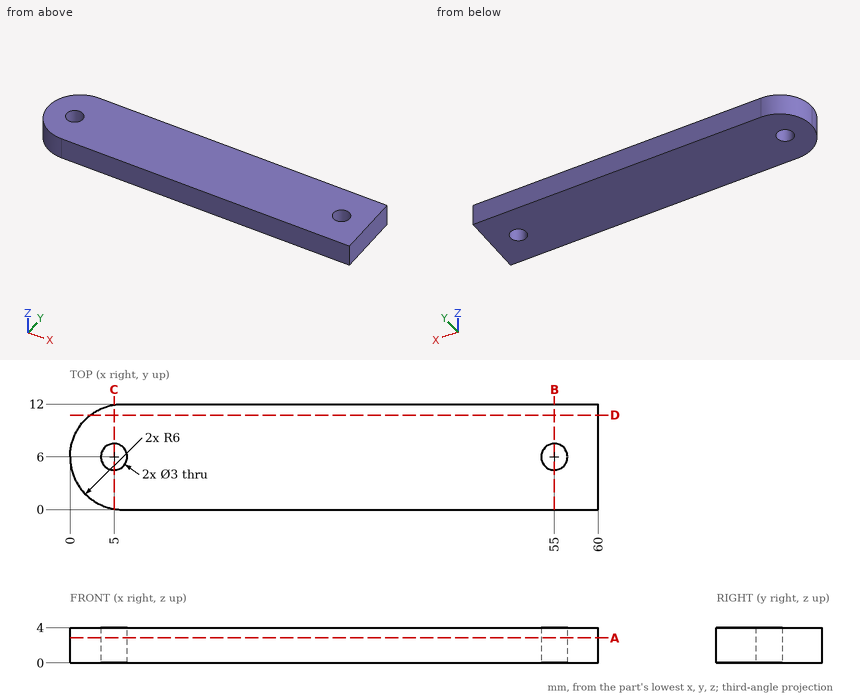
Here's the drawing with two shaded views (mm, measured from the low corner). I have some questions. Coordinates: 2 decimals unless noted, no trailing zeros. Write each loop counter-clockwise with the first axis right and the second up, starting at its lowest first coordinate (ties: lowest second). Pieces come first, ordered by that corner, then holes. Notation, with made-up numbers: (16, -2) -> (55, -2) arc R23 ccw to (55, 35) -> close; hole circle Ø11 at (37, -23.75). An arc over 180 degrees is marked (long way). One line per question, with ' | ' between items. Start each with the question number.
1. If we section it at C-C (x = 5): Please give me the cut outline in (y, z), and give its area (3 significant figures).
2. If we section it at B-B (x = 55): Please give me the cut outline in (y, z), and give its area (3 significant figures).
3. Please list where these lines run through material, in increasing order: line 1 along Y through (x, z) = (55, 2.5); line 2 along X through (y, z) = (5, 3.5); line 3 along Y through (x, z) = (6, 2.85).
4. Will this pin go through, and if not, where does the flat tip stop? P1, Ø2, axis at y = 9.5, z = 1.5, coming from the -X side.
5. If we section it at A-A (z = 2.85): Count the separate pieces of the cut face and the enclosed holes in it, and give its area (3 significant figures).
6. If we section it at D-D (y = 10.75): Please give me the cut outline in (x, z), and give its area (3 significant figures).
Return value:
1) outline: (0.08, 0) -> (4.5, 0) -> (4.5, 4) -> (0.08, 4) -> close; (7.5, 0) -> (11.92, 0) -> (11.92, 4) -> (7.5, 4) -> close | area: 35.3 mm²
2) outline: (0, 0) -> (4.5, 0) -> (4.5, 4) -> (0, 4) -> close; (7.5, 0) -> (12, 0) -> (12, 4) -> (7.5, 4) -> close | area: 36.0 mm²
3) line 1: y = 0 to 4.5, 7.5 to 12 | line 2: x = 0.08 to 3.88, 6.12 to 53.88, 56.12 to 60 | line 3: y = 0 to 4.88, 7.12 to 12
4) P1: stops at x = 0.55
5) separate pieces: 1 | enclosed holes: 2 | area: 690 mm²
6) outline: (2.33, 0) -> (60, 0) -> (60, 4) -> (2.33, 4) -> close | area: 231 mm²
